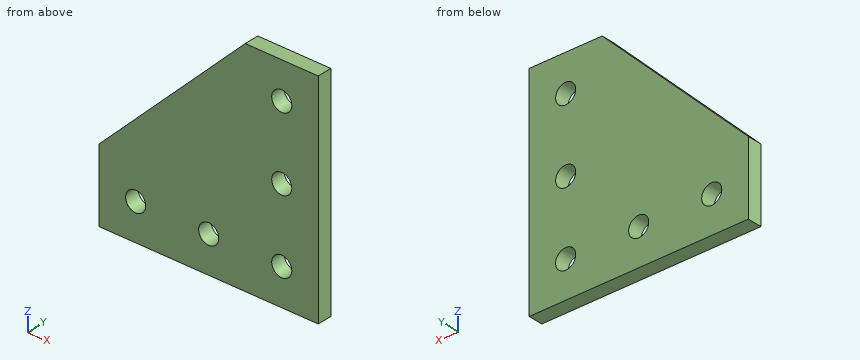
Autodesk Inventor part; units mm, degrees
ref_plane "YZ Plane" through (0, 0, 0) normal (1, 0, 0) x (0, 1, 0)
ref_plane "XZ Plane" through (0, 0, 0) normal (0, 1, 0) x (-1, 0, 0)
ref_plane "XY Plane" through (0, 0, 0) normal (0, 0, 1) x (1, 0, 0)
sketch "Sketch1" plane through (0, 0, 0) normal (0, 1, 0) x (-1, 0, 0)
  line L0 (-30, 30) -> (-10, 30)
  line L1 (30, -10) -> (30, -30)
  line L2 (30, -30) -> (-30, -30)
  line L3 (-30, -30) -> (-30, 30)
  line L4 (-30, 30) -> (30, -30) construction
  line L5 (30, 30) -> (-30, -30) construction
  line L6 (-30, 30) -> (-10, 30)
  line L7 (-10, -30) -> (-30, -30)
  line L8 (-30, -30) -> (-30, 30)
  line L9 (30, -30) -> (-10, -30)
  line L10 (30, -10) -> (30, -30)
  line L11 (-10, 30) -> (30, -10)
  circle A0 centre (-20, -20) radius 2.75
  circle A1 centre (-20, 0) radius 2.75
  circle A2 centre (-20, 20) radius 2.75
  circle A3 centre (0, -20) radius 2.75
  circle A4 centre (20, -20) radius 2.75
  point P0 (0, 0)
  dimension "d0" = 60
  dimension "d1" = 60
  dimension "d4" = 5.5
  dimension "d5" = 5.5
  dimension "d6" = 5.5
  dimension "d7" = 5.5
  dimension "d8" = 5.5
extrude "Extrusion1" add sketch "Sketch1" along normal blind 4
properties part number "2020-90-plate"
Could you check a few things on this model? Use its own coordinates, in mm. Give positions to 0.01 mm unless a question says otherwise; leave off trailing zeros. Order: outer loops, then holes, each group sorted by start corner. A loop starts at its lowest first (then second) coordinate and runs counter-clockwise, first axis right, second up. Notation, with made-up numbers: (49.5, 77) - (94.5, 77) arc R13 cw to (94.5, 97) - close; hole circle Ø8 at (43, -35). An arc over 180 degrees is marked (long way). Return JSON: item names as keys, results as strings. Group by question number.
Q1. Will this pin go through, and if not, where does the flat tip stop? pin 1 Ø1 at (x, z) = (-18, -14.5) entering from -Y.
Q2. Suppose I cut it at C-C, the plane z = -22. Please give me the cut outline in (x, y), and give its area (3 significant figures).
Q3. Suppose I cut it at B-B, the plane x = 0. Please give me the cut outline in (y, z), and give its area (3 significant figures).
Q4. Suppose I cut it at D-D, the plane x = 6.5. Please give me the cut outline in (y, z), and give its area (3 significant figures).
Q5. Please list where these lines run through material, in increasing order: line 1 along Z through (x, y) = (20, 1); line 2 along X through (y, z) = (1.1, -18); line 3 along Z through (x, y) = (-25, 2.95). Write a range as [from, to].
Resolved:
{
 "1": {"pin 1": "stops at y = 0"},
 "2": {"outline": "(-30, 0) - (-21.89, 0) - (-21.89, 4) - (-30, 4) - close; (-18.11, 0) - (-1.89, 0) - (-1.89, 4) - (-18.11, 4) - close; (1.89, 0) - (18.11, 0) - (18.11, 4) - (1.89, 4) - close; (21.89, 0) - (30, 0) - (30, 4) - (21.89, 4) - close", "area": "195 mm2"},
 "3": {"outline": "(0, -30) - (4, -30) - (4, -22.75) - (0, -22.75) - close; (0, -17.25) - (4, -17.25) - (4, 20) - (0, 20) - close", "area": "178 mm2"},
 "4": {"outline": "(0, -30) - (4, -30) - (4, 26.5) - (0, 26.5) - close", "area": "226 mm2"},
 "5": {"line 1": "z = [-30, -22.75], [-17.25, -2.75], [2.75, 17.25], [22.75, 30]", "line 2": "x = [-30, -21.89], [-18.11, -1.89], [1.89, 18.11], [21.89, 30]", "line 3": "z = [-30, -5]"}
}
